Source: CAD feature listing. Evaluate the final solid. Frame: model axes, mm. Face numbers are marked on the shaded views. A direction names the side the tool comes from. Round coordinates to 2 decimals unless told otherwise and drop trailing zeros. Write each loop counter-clockwise with the first axis right and the second up, starting at its lowest first coordinate (ties: lowest second). Pieces come first, ordered by that corner, then holes. Notation, with made-up numbers: M 77.5,28.25 L 121.5,28.25 A14 ccw 121.5,45.25 Z; hole C -27,35 d8. An arc over 180 degrees is marked long. Answer in a Markdown table with one row per item.
from build123d import *

# Parameters (mm, degrees)
F0_W     = 48
F0_H     = 50.5
F1_DEPTH = 13.5
F2_W     = 45
F2_H     = 47.5
F3_DEPTH = 12
F4_R     = 5


with BuildPart() as f1:
    # F0 (on Top) → F1 (new body)
    with BuildSketch(Plane.XY):
        Rectangle(F0_W, F0_H)
    extrude(amount=F1_DEPTH)

    # F2 (on face) → F3 (cut)
    with BuildSketch(Plane.XY.offset(13.5)):
        Rectangle(F2_W, F2_H)
    extrude(amount=-F3_DEPTH, mode=Mode.SUBTRACT)

    # F4
    f4_edges = [f1.edges().sort_by_distance(p)[0] for p in [
        (22.5, 23.75, 7.5),
        (-22.5, 23.75, 7.5),
        (22.5, -23.75, 7.5),
        (-22.5, -23.75, 7.5),
        (-24, -25.25, 6.75),
        (24, -25.25, 6.75),
        (-24, 25.25, 6.75),
        (24, 25.25, 6.75),
    ]]
    fillet(f4_edges, radius=F4_R)


solid = f1.part
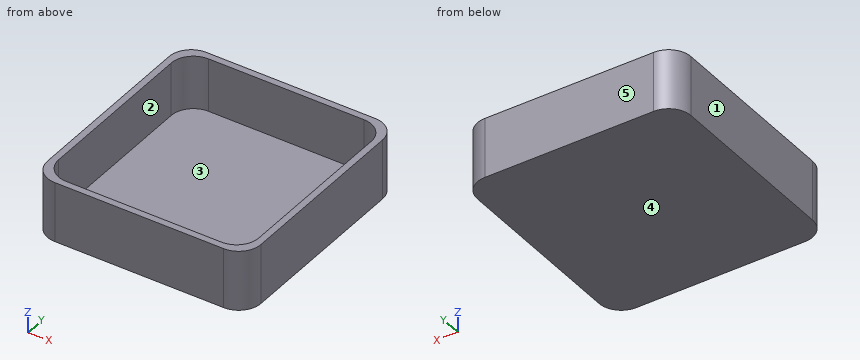
Q1. Section A-A (z = 7.5). Return loops of the section in (x, y).
Solutions:
| item | result |
|---|---|
| outline | M -24,-20.25 A5 ccw -19,-25.25 L 19,-25.25 A5 ccw 24,-20.25 L 24,20.25 A5 ccw 19,25.25 L -19,25.25 A5 ccw -24,20.25 Z; hole M -22.5,-18.75 A5 ccw -17.5,-23.75 L 17.5,-23.75 A5 ccw 22.5,-18.75 L 22.5,18.75 A5 ccw 17.5,23.75 L -17.5,23.75 A5 ccw -22.5,18.75 Z |
Q2. Access query for the marked faces 1 and 2. Directions: +Z, -Z, +X, -X, +Y, -Y. A direction counts if a zero-diameter tool reaches every point of the face in a straight line with its end or side. Return the directions, or none.
Solutions:
| item | result |
|---|---|
| face 1 | +Z, -Z, -X, +Y, -Y |
| face 2 | +Z |
Q3. Section B-B (y = -17.5). Return loops of the section in (x, z), and give its area (3 significant figures).
Solutions:
| item | result |
|---|---|
| outline | M -24,0 L 24,0 L 24,13.5 L 22.5,13.5 L 22.5,1.5 L -22.5,1.5 L -22.5,13.5 L -24,13.5 Z |
| area | 108 mm2 |
Q4. Contact query for flat-ended pins moving along their axis: pin 1 Ø6 at (x, y) = (1, 7.5) entering from -Z; pin 2 Ø13.5 at (x, y) = (-9.5, -11) entering from +Z. Output: stop coordinate, or through.
Solutions:
| item | result |
|---|---|
| pin 1 | stops at z = 0 |
| pin 2 | stops at z = 1.5 |
Q5. Material intervals for probe 1 along Y at (x, z) = (-3.5, 5.5); probe 2 along X at (y, z) = (9.5, 7); probe 3 along Z at (x, y) = (-6, 5.5), sorted ascending.
Solutions:
| item | result |
|---|---|
| probe 1 | y = -25.25 to -23.75, 23.75 to 25.25 |
| probe 2 | x = -24 to -22.5, 22.5 to 24 |
| probe 3 | z = 0 to 1.5 |
Q6. Section C-C (x = -6). Return loops of the section in (y, z), and give its area (3 significant figures).
Solutions:
| item | result |
|---|---|
| outline | M -25.25,0 L 25.25,0 L 25.25,13.5 L 23.75,13.5 L 23.75,1.5 L -23.75,1.5 L -23.75,13.5 L -25.25,13.5 Z |
| area | 112 mm2 |
Q7. Pull-direction query (Z, two-part tool) for the marked faces 3, 4 and 5; classes: pulls with the +Z half, pulls with the -Z half, needs draft (parallel to the pull), parting line crosses it, or undercut.
Solutions:
| item | result |
|---|---|
| face 3 | pulls with the +Z half |
| face 4 | pulls with the -Z half |
| face 5 | needs draft |
